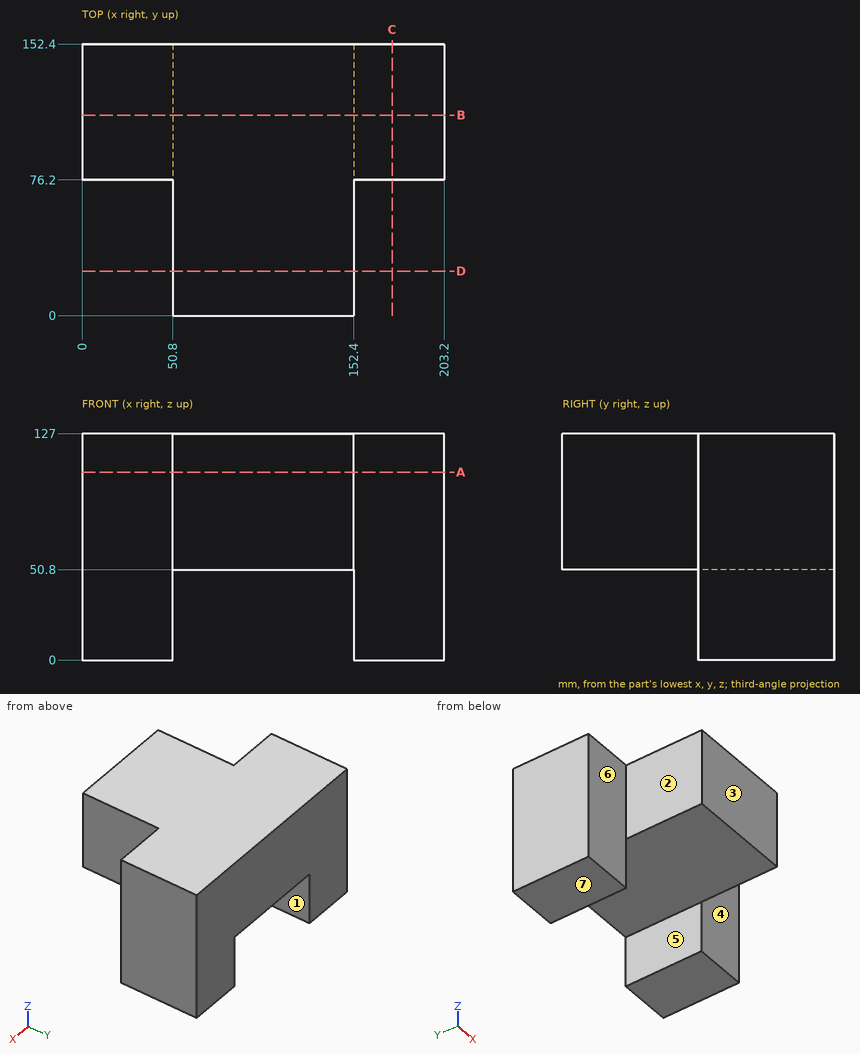
The figure shows three views and two pictorial views of one solid part (mm, origin at its lowest corner). Answer the questions. A direction names the side the tool comes from. Coordinates: 2 decimals unless noted, no trailing zeros. Write each loop counter-clockwise with the first axis right and the second up, starting at its lowest first coordinate (ties: lowest second). Pieces come first, ordered by that corner, then holes.
1. The part is cut by section B-B, the plane y = 112.5. Write down the section's boundary in (x, z).
Results list:
outline: (0, 0) - (50.8, 0) - (50.8, 50.8) - (152.4, 50.8) - (152.4, 0) - (203.2, 0) - (203.2, 127) - (0, 127) - close
2. The part is cut by section A-A, the plane z = 105.5. Write down the section's boundary in (x, y), and give its area (3 significant figures).
Results list:
outline: (0, 76.2) - (50.8, 76.2) - (50.8, 0) - (152.4, 0) - (152.4, 76.2) - (203.2, 76.2) - (203.2, 152.4) - (0, 152.4) - close
area: 23,200 mm2
3. The part is cut by section D-D, the plane y = 25. Write down the section's boundary in (x, z), and give its area (3 significant figures).
Results list:
outline: (50.8, 50.8) - (152.4, 50.8) - (152.4, 127) - (50.8, 127) - close
area: 7,740 mm2
4. For a pull along X with two mould halves and no side action, classify the marked faces 1, 2 and 3 as +X half, -X half, draft (parallel to the pull), parting line (faces both ways), or undercut.
Results list:
face 1: undercut
face 2: -X half
face 3: draft
5. Consider line 1 along X through (y, z) = (144.5, 42); line 2 along Z through (x, y) = (136, 55); line 3 along Y through (x, z) = (195, 97). Determine where each line is inside the solid, lowest interval first.
Results list:
line 1: x = 0 to 50.8, 152.4 to 203.2
line 2: z = 50.8 to 127
line 3: y = 76.2 to 152.4
6. The part is cut by section C-C, the plane x = 174. Write down the section's boundary in (y, z).
Results list:
outline: (76.2, 0) - (152.4, 0) - (152.4, 127) - (76.2, 127) - close
7. For the marked faces 4, 5, 6 and 7, determine the directions among +Z, -Z, +X, -X, +Y, -Y from which every point of the face is accessible in a straight line to the end or side of a thin tool.
Results list:
face 4: +Z, -Z, +X, -Y
face 5: -Z, +Y, -Y
face 6: +Z, -Z, -X, -Y
face 7: -Z, +X, -X, +Y, -Y
8. A flat-ended cylindrical pin translates along its axis: pin 1 (1.5 mm diameter, centred on x = 177, z = 22.5, fed in from -Y). Find the tip coordinate at first contact, or state that the pin passes through.
Results list:
pin 1: stops at y = 76.2
